Read the model definition and answer for the solid it produces. Units are mm, in the model's axes. Coordinates: 2 decimals unless noted, no trailing zeros. Write each loop counter-clockwise with the first axis right and the second up, starting at its lowest first coordinate (ties: lowest second). Pieces come first, ordered by that corner, then holes. Notation, with made-up numbers: (46, 0.5) -> (104, 0.5) arc R13 cw to (104, 19.5) -> close; hole circle Ø5 at (13.5, 70). An arc over 180 degrees is marked (long way). Return JSON: item names as keys, results as strings.
from build123d import *

# Parameters (mm, degrees)
SKETCH1_W           = 75
SKETCH1_H           = 13
BOSS_EXTRUDE1_DEPTH = 13


with BuildPart() as part:
    # Sketch1 → Boss-Extrude1 (new body)
    with BuildSketch(Plane(origin=(0, 0, 0), x_dir=(1, 0, 0), z_dir=(0, 1, 0))):
        Rectangle(SKETCH1_W, SKETCH1_H)
        with BuildLine():
            ThreePointArc((0, 3.801315562), (-8.5, 0), (0, -3.801315562))
            ThreePointArc((0, -3.801315562), (8.5, 0), (0, 3.801315562))
        make_face(mode=Mode.SUBTRACT)
    extrude(amount=BOSS_EXTRUDE1_DEPTH)


solid = part.part
1. Consider L1, parallel to Z at x = -3.4, y = 6.5; L2, parallel to X at y = 5.5, z = 4.5; L3, parallel to X at y = 9.5, z = 4.25. Determine where each line is inside the solid, lowest interval first.
Taken from the geometry:
{"L1": "z = -6.5 to -5.1, 5.1 to 6.5", "L2": "x = -37.5 to -5.8, -1 to 1, 5.8 to 37.5", "L3": "x = -37.5 to -6.22, -0.58 to 0.58, 6.22 to 37.5"}
2. For a pull along Z with two mould halves and no side action, classify faces 1 (the face through (-1, 6, -6.5)), 2 (the face through (-8.497, 6.409, -0.164)), 3 (the face through (-0.5, 0, -4.4)) as +Z half, -Z half, draft (parallel to the pull), parting line (faces both ways), or undercut.
Taken from the geometry:
{"face 1": "-Z half", "face 2": "undercut", "face 3": "draft"}
3. The part is cut by section A-A (x = 3.4). Determine the outline of the cut face in (y, z), then the cut area to 3 significant figures.
Taken from the geometry:
{"outline": "(0, -6.5) -> (13, -6.5) -> (13, -5.1) -> (0, -5.1) -> close; (0, 5.1) -> (13, 5.1) -> (13, 6.5) -> (0, 6.5) -> close", "area": "36.4 mm2"}
4. The part is cut by section B-B (z = 0). Determine the outline of the cut face in (x, y), then the cut area to 3 significant figures.
Taken from the geometry:
{"outline": "(-37.5, 0) -> (-8.5, 0) -> (-8.5, 13) -> (-37.5, 13) -> close; (8.5, 0) -> (37.5, 0) -> (37.5, 13) -> (8.5, 13) -> close", "area": "754 mm2"}
5. The part is cut by section C-C (y = 2.25). Determine the outline of the cut face in (x, z), then the cut area to 3 significant figures.
Taken from the geometry:
{"outline": "(-37.5, -6.5) -> (37.5, -6.5) -> (37.5, 6.5) -> (-37.5, 6.5) -> close; hole (0, -3.8) arc R5.1 ccw (long way) to (0, 3.8) arc R5.1 ccw (long way) to start", "area": "829 mm2"}
